Input: dimensioned drawing with shaded views. Units: mm. Origin: part minimum x, y, z. Coordinates: 2 decimals unless noted, no trailing zeros. Loops run counter-clockwise (first coordinate to the right, second up) from the corner with the lowest first, then second, coordinate; pieces in that order, holes last.
Item 1: Line query: probe 1 along X at (y, z) = (1.2, 42.5) (1 decimal); probe 2 along Z at (x, y) = (2.9, 1.8) (1 decimal); probe 3 along X at (y, z) = (0.95, 17.5) (1 decimal). Output: solid intervals per line, ascending.
Item 2: Section query A-A, the plane x = 2.9. Return the cut outline in (y, z) (1 decimal).
Item 3: Pin query (flat end, axial travel): pin 1 Ø1 at (x, y) = (46.5, 0.5) entering from -Z; pin 2 Ø1.8 at (x, z) = (57.04, 18.76) entering from -Y. Return the tip coordinate at first contact, or that it passes through.
Item 4: Section query D-D, the plane z = 48. Return the cut outline in (x, y).
Item 5: Section query C-C, the plane z = 2.9. Return the cut outline in (x, y) (1 decimal).
Item 6: Section query B-B, the plane y = 2. State how many separate pieces and enclosed holes the cut face has, then the cut area to 3 significant figures.
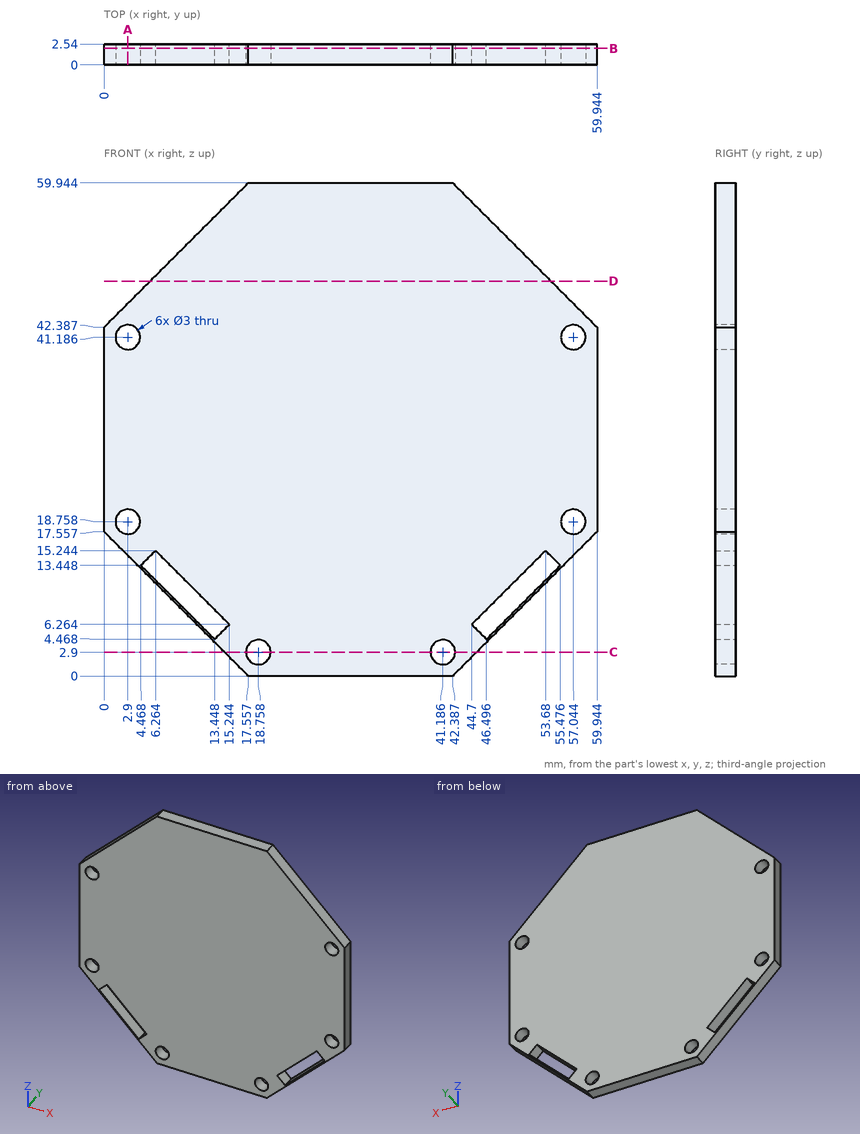
Verdict:
1. probe 1: x = 0.1 to 2.2, 3.6 to 56.3, 57.8 to 59.8
1. probe 2: z = 14.7 to 17.3, 20.3 to 39.7, 42.7 to 45.3
1. probe 3: x = 0.1 to 2.1, 3.7 to 56.2, 57.9 to 59.9
2. outline: (0, 14.7) - (2.5, 14.7) - (2.5, 17.3) - (0, 17.3) - close; (0, 20.3) - (2.5, 20.3) - (2.5, 39.7) - (0, 39.7) - close; (0, 42.7) - (2.5, 42.7) - (2.5, 45.3) - (0, 45.3) - close
3. pin 1: stops at z = 3.61
3. pin 2: passes through
4. outline: (5.61, 0) - (54.33, 0) - (54.33, 2.54) - (5.61, 2.54) - close
5. outline: (14.7, 0) - (17.3, 0) - (17.3, 2.5) - (14.7, 2.5) - close; (20.3, 0) - (39.7, 0) - (39.7, 2.5) - (20.3, 2.5) - close; (42.7, 0) - (45.3, 0) - (45.3, 2.5) - (42.7, 2.5) - close
6. separate pieces: 1
6. enclosed holes: 8
6. area: 2,870 mm2
